from build123d import *

# Parameters (mm, degrees)
EXTRUDE_THIN1_OUTLINE_W     = 97
EXTRUDE_THIN1_OUTLINE_H     = 101.4
EXTRUDE_THIN1_DEPTH         = 2.4
EXTRUDE_THIN1_START         = 8.1
EXTRUDE_THIN1_2_OUTLINE_W   = 97
EXTRUDE_THIN1_2_OUTLINE_H   = 101.4
EXTRUDE_THIN1_2_DEPTH       = 2.4
EXTRUDE_THIN1_START_2       = 2.4
EXTRUDE_THIN1_3_OUTLINE_W   = 97
EXTRUDE_THIN1_3_OUTLINE_H   = 101.4
EXTRUDE_THIN1_3_OUTLINE_W_2 = 92.2
EXTRUDE_THIN1_3_OUTLINE_H_2 = 96.6
EXTRUDE_THIN1_3_DEPTH       = 5.7
SKETCH4_W                   = 92.2
SKETCH4_H                   = 96.6
CUT_EXTRUDE2_DEPTH          = 2.4
SKETCH5_R                   = 4.5
BOSS_EXTRUDE1_DEPTH         = 8
SKETCH7_R                   = 1.5
CUT_EXTRUDE3_DEPTH          = 13.4
SKETCH10_R                  = 3
CUT_EXTRUDE4_DEPTH          = 3
SKETCH11_R                  = 3
CUT_EXTRUDE5_DEPTH          = 0.8
SKETCH12_W                  = 97
SKETCH12_H                  = 101.4
SKETCH12_W_2                = 94.6
SKETCH12_H_2                = 99
CUT_EXTRUDE_THIN2_DEPTH     = 3
FILLET2_R                   = 3.2
FILLET3_R                   = 2.4
FILLET4_R                   = 2.3


# Read off the part's stored shape, not the designer's step: Extrude-Thin1
with BuildPart() as part:
    # Extrude-Thin1 outline → Extrude-Thin1 (new body)
    with BuildSketch(Plane.XY):
        Rectangle(EXTRUDE_THIN1_OUTLINE_W, EXTRUDE_THIN1_OUTLINE_H)
    extrude(amount=EXTRUDE_THIN1_DEPTH)



with BuildPart() as body_2:
    # Extrude-Thin1 2 outline → Extrude-Thin1 2 (new body)
    with BuildSketch(Plane.XY.offset(EXTRUDE_THIN1_START)):
        Rectangle(EXTRUDE_THIN1_2_OUTLINE_W, EXTRUDE_THIN1_2_OUTLINE_H)
    extrude(amount=EXTRUDE_THIN1_2_DEPTH)


with BuildPart() as part_1:
    add(part.part)

    add(body_2.part)  # Extrude-Thin1 3 merges body 2
    # Extrude-Thin1 3 outline → Extrude-Thin1 3 (add)
    with BuildSketch(Plane.XY.offset(EXTRUDE_THIN1_START_2)):
        Rectangle(EXTRUDE_THIN1_3_OUTLINE_W, EXTRUDE_THIN1_3_OUTLINE_H)
        Rectangle(EXTRUDE_THIN1_3_OUTLINE_W_2, EXTRUDE_THIN1_3_OUTLINE_H_2, mode=Mode.SUBTRACT)
    extrude(amount=EXTRUDE_THIN1_3_DEPTH)

    # Sketch4 → Cut-Extrude2 (cut)
    with BuildSketch(Plane.XY.offset(10.5)):
        Rectangle(SKETCH4_W, SKETCH4_H)
    extrude(amount=-CUT_EXTRUDE2_DEPTH, mode=Mode.SUBTRACT)

    # Sketch5 → Boss-Extrude1 (add)
    with BuildSketch(Plane.XY.offset(2.4)):
        with Locations((-40.98, 42.8)):
            Circle(SKETCH5_R)
        with Locations((40.98, 42.8)):
            Circle(SKETCH5_R)
        with Locations((40.98, -42.8)):
            Circle(SKETCH5_R)
        with Locations((-40.98, -42.8)):
            Circle(SKETCH5_R)
    extrude(amount=BOSS_EXTRUDE1_DEPTH)

    # Sketch7 → Cut-Extrude3 (cut)
    with BuildSketch(Plane.XY.offset(10.4)):
        with Locations((-40.98, 42.8)):
            Circle(SKETCH7_R)
        with Locations((40.98, 42.8)):
            Circle(SKETCH7_R)
        with Locations((40.98, -42.8)):
            Circle(SKETCH7_R)
        with Locations((-40.98, -42.8)):
            Circle(SKETCH7_R)
    extrude(amount=-CUT_EXTRUDE3_DEPTH, mode=Mode.SUBTRACT)

    # Sketch10 → Cut-Extrude4 (cut)
    with BuildSketch(Plane(origin=(0, 0, 0), x_dir=(-1, 0, 0), z_dir=(0, 0, -1))):
        with Locations((-40.98, 42.8)):
            Circle(SKETCH10_R)
        with Locations((40.98, 42.8)):
            Circle(SKETCH10_R)
        with Locations((40.98, -42.8)):
            Circle(SKETCH10_R)
        with Locations((-40.98, -42.8)):
            Circle(SKETCH10_R)
    extrude(amount=-CUT_EXTRUDE4_DEPTH, mode=Mode.SUBTRACT)

    # Sketch11 → Cut-Extrude5 (cut)
    with BuildSketch(Plane(origin=(0, 0, 0), x_dir=(-1, 0, 0), z_dir=(0, 0, -1))):
        with Locations((-40.98, -35.8)):
            Circle(SKETCH11_R)
        with Locations((40.98, -35.8)):
            Circle(SKETCH11_R)
        with Locations((40.98, 35.8)):
            Circle(SKETCH11_R)
        with Locations((-40.98, 35.8)):
            Circle(SKETCH11_R)
    extrude(amount=-CUT_EXTRUDE5_DEPTH, mode=Mode.SUBTRACT)

    # Sketch12 → Cut-Extrude-Thin2 (cut)
    with BuildSketch(Plane.XY.offset(10.5)):
        Rectangle(SKETCH12_W, SKETCH12_H)
        Rectangle(SKETCH12_W_2, SKETCH12_H_2, mode=Mode.SUBTRACT)
    extrude(amount=-CUT_EXTRUDE_THIN2_DEPTH, mode=Mode.SUBTRACT)

    # Fillet2
    fillet2_edges = [part_1.edges().sort_by_distance(p)[0] for p in [
        (48.5, -50.7, 3.75),
        (-48.5, -50.7, 3.75),
        (-48.5, 50.7, 3.75),
        (48.5, 50.7, 3.75),
    ]]
    fillet(fillet2_edges, radius=FILLET2_R)

    # Fillet3
    fillet3_edges = [part_1.edges().sort_by_distance(p)[0] for p in [
        (-47.3, 49.5, 9),
        (47.3, 49.5, 9),
        (47.3, -49.5, 9),
        (-47.3, -49.5, 9),
    ]]
    fillet(fillet3_edges, radius=FILLET3_R)

    # Fillet4
    # the kernel refuses this fillet: 2.3 mm, written as the material it adds along each edge
    with BuildSketch(Plane(origin=(-40.98, 42.8, 2.4), x_dir=(1, 0, 0), z_dir=(0, -1, 0))) as fillet4_piece_1:
        with BuildLine():
            CenterArc((4.5 + FILLET4_R, FILLET4_R), FILLET4_R, 180, 90)
            Line((4.5, FILLET4_R), (4.5, 0))
            Line((4.5, 0), (4.5 + FILLET4_R, 0))
        make_face()
    revolve(axis=Axis((-40.98, 42.8, 2.4), (0, 0, 1)))
    with BuildSketch(Plane(origin=(40.98, 42.8, 2.4), x_dir=(1, 0, 0), z_dir=(0, -1, 0))) as fillet4_piece_2:
        with BuildLine():
            CenterArc((4.5 + FILLET4_R, FILLET4_R), FILLET4_R, 180, 90)
            Line((4.5, FILLET4_R), (4.5, 0))
            Line((4.5, 0), (4.5 + FILLET4_R, 0))
        make_face()
    revolve(axis=Axis((40.98, 42.8, 2.4), (0, 0, 1)))
    with BuildSketch(Plane(origin=(40.98, -42.8, 2.4), x_dir=(1, 0, 0), z_dir=(0, -1, 0))) as fillet4_piece_3:
        with BuildLine():
            CenterArc((4.5 + FILLET4_R, FILLET4_R), FILLET4_R, 180, 90)
            Line((4.5, FILLET4_R), (4.5, 0))
            Line((4.5, 0), (4.5 + FILLET4_R, 0))
        make_face()
    revolve(axis=Axis((40.98, -42.8, 2.4), (0, 0, 1)))
    with BuildSketch(Plane(origin=(-40.98, -42.8, 2.4), x_dir=(1, 0, 0), z_dir=(0, -1, 0))) as fillet4_piece_4:
        with BuildLine():
            CenterArc((4.5 + FILLET4_R, FILLET4_R), FILLET4_R, 180, 90)
            Line((4.5, FILLET4_R), (4.5, 0))
            Line((4.5, 0), (4.5 + FILLET4_R, 0))
        make_face()
    revolve(axis=Axis((-40.98, -42.8, 2.4), (0, 0, 1)))


solid = part_1.part
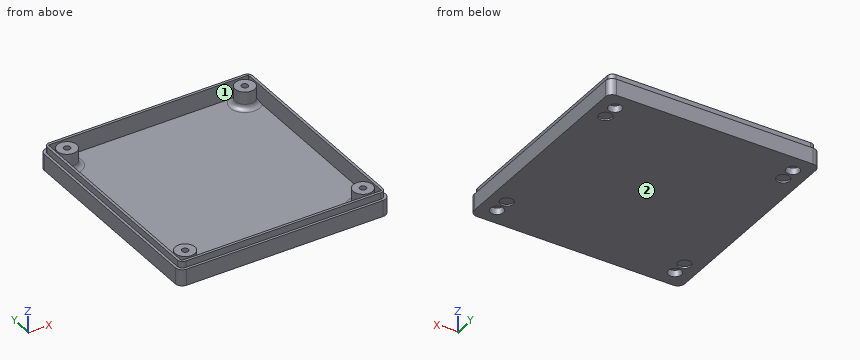
Here's how the part is built. I have some questions about the finished solid (model axes, mm). Face numbers are marked on the shaded views. Round coordinates to 2 decimals unless told otherwise and drop trailing zeros. Write each loop counter-clockwise with the first axis right and the second up, starting at its lowest first coordinate (ties: lowest second). Pieces come first, ordered by that corner, then holes.
1. Suppose I cut it at C-C (y = -23). List the corners of the cut face in (x, z) for me.
2. Suppose I cut it at B-B (x = -14.5). List the corners of the cut face in (y, z) for me, and give its area (3 significant figures).
3. If we mould it in two halves opening along Y, with no side actions, what happens to the marked faces 1 and 2? For each: released by +Y, released by -Y, zero draft, split by the parting line, or undercut.
4. I need wall thicknesses on L1, parallel to Y at x = 40.98, z = 0.45; L2, parallel to X at y = 43, z = 9.75; L3, parallel to Y at x = -40.98, z = 1.7. Which ranges of each line are inside material? Lowest first, please.
5. Suppose I cut it at A-A (z = 6). State how many separate pieces and enclosed holes the cut face has, and give its area (3 significant figures).
6. Will these pins go through, and if not, where does the flat tip stop? pin 1 Ø1.1 at (x, y) = (-45.5, 47.5) entering from +Z; pin 2 Ø5 at (x, y) = (40.98, -35.8) entering from -Z; pin 3 Ø4.5 at (x, y) = (-41, -42) entering from +Z.
Answer sheet:
1. outline: (-48.5, 0) - (48.5, 0) - (48.5, 7.5) - (47.3, 7.5) - (47.3, 10.5) - (46.1, 10.5) - (46.1, 2.4) - (-46.1, 2.4) - (-46.1, 10.5) - (-47.3, 10.5) - (-47.3, 7.5) - (-48.5, 7.5) - close
2. outline: (-50.7, 0) - (50.7, 0) - (50.7, 7.5) - (49.5, 7.5) - (49.5, 10.5) - (48.3, 10.5) - (48.3, 2.4) - (-48.3, 2.4) - (-48.3, 10.5) - (-49.5, 10.5) - (-49.5, 7.5) - (-50.7, 7.5) - close
2. area: 275 mm2
3. face 1: undercut
3. face 2: zero draft
4. L1: y = -50.7 to -45.8, -39.8 to -38.8, -32.8 to 32.8, 38.8 to 39.8, 45.8 to 50.7
4. L2: x = -47.3 to -46.1, -45.48 to -42.47, -39.49 to -36.48, 36.48 to 39.49, 42.47 to 45.48, 46.1 to 47.3
4. L3: y = -50.7 to -45.8, -39.8 to 39.8, 45.8 to 50.7
5. separate pieces: 5
5. enclosed holes: 5
5. area: 1,150 mm2
6. pin 1: stops at z = 2.55
6. pin 2: stops at z = 0.8
6. pin 3: stops at z = 10.4
